```python
from build123d import *

# Parameters (mm, degrees)
F1_DEPTH  = 35
F2_R      = 3
F3_DEPTH  = 34.3740698971
F4_R      = 5
F5_DEPTH  = 120.001
F6_R      = 11.25
F7_DEPTH  = 7.5
F8_R      = 11.25
F9_DEPTH  = 7.5
F10_R     = 11.25
F11_DEPTH = 47.5
F12_R     = 11.25
F13_DEPTH = 47.5
F14_R     = 2.05
F15_DEPTH = 60
F16_R     = 3.5
F17_DEPTH = 15
F18_R     = 5


with BuildPart() as f1:
    # F0 (on Front) → F1 (new body)
    with BuildSketch(Plane.XZ):
        with BuildLine():
            Line((-40, 19.3730698971), (-60, 5))
            Line((-60, 5), (-60, 0))
            Line((-60, 0), (-60, -100))
            Line((-60, -100), (-40, -100))
            Line((-40, -100), (-30, -15))
            Line((-30, -15), (0, -15))
            Line((0, -15), (30, -15))
            Line((30, -15), (40, -100))
            Line((40, -100), (60, -100))
            Line((60, -100), (60, 0))
            Line((60, 0), (60, 5))
            Line((60, 5), (40, 19.3730698971))
            Line((40, 19.3730698971), (10, 19.3730698971))
            ThreePointArc((10, 19.3730698971), (0, 9.3730698971), (-10, 19.3730698971))
            Line((-10, 19.3730698971), (-40, 19.3730698971))
        make_face()
    extrude(amount=F1_DEPTH)

    # F2 (on face) → F3 (cut, through all)
    with BuildSketch(Plane(origin=(0, 0, -15), x_dir=(1, 0, 0), z_dir=(0, 0, -1))):
        with Locations((-16.9, 17.5)):
            Circle(F2_R)
        with Locations((16.9, 17.5)):
            Circle(F2_R)
    extrude(amount=-F3_DEPTH, mode=Mode.SUBTRACT)

    # F4 (on face) → F5 (cut, through all)
    with BuildSketch(Plane(origin=(-60, 0, 0), x_dir=(0, -1, 0), z_dir=(-1, 0, 0))):
        with Locations((17.5, -85)):
            Circle(F4_R)
    extrude(amount=-F5_DEPTH, mode=Mode.SUBTRACT)

    # F6 (on face) → F7 (cut)
    with BuildSketch(Plane(origin=(-60, 0, 0), x_dir=(0, -1, 0), z_dir=(-1, 0, 0))):
        with Locations((17.5, -85)):
            Circle(F6_R)
    extrude(amount=-F7_DEPTH, mode=Mode.SUBTRACT)

    # F8 (on face) → F9 (cut)
    with BuildSketch(Plane.YZ.offset(60)):
        with Locations((-17.5, -85)):
            Circle(F8_R)
    extrude(amount=-F9_DEPTH, mode=Mode.SUBTRACT)

    # F10 (on Right) → F11 (cut)
    with BuildSketch(Plane.YZ):
        with Locations((-17.5, -85)):
            Circle(F10_R)
    extrude(amount=-F11_DEPTH, mode=Mode.SUBTRACT)

    # F12 (on Right) → F13 (cut)
    with BuildSketch(Plane.YZ):
        with Locations((-17.5, -85)):
            Circle(F12_R)
    extrude(amount=F13_DEPTH, mode=Mode.SUBTRACT)

    # F14 (on Top) → F15 (cut, symmetric)
    with BuildSketch(Plane.XY):
        with Locations((-47, -18)):
            Circle(F14_R)
        with Locations((47, -18)):
            Circle(F14_R)
    extrude(amount=F15_DEPTH, both=True, mode=Mode.SUBTRACT)

    # F16 (on face) → F17 (cut)
    with BuildSketch(Plane.XY.offset(19.3730698971)):
        with Locations((-47, -18)):
            Circle(F16_R)
        with Locations((47, -18)):
            Circle(F16_R)
    extrude(amount=-F17_DEPTH, mode=Mode.SUBTRACT)

    # F18
    f18_edges = [f1.edges().sort_by_distance(p)[0] for p in [
        (60, -35, -47.5),
        (60, 0, -47.5),
        (-60, -35, -47.5),
        (-60, 0, -47.5),
        (-50, 0, 12.186535),
        (-50, -35, 12.186535),
        (50, -35, 12.186535),
        (50, 0, 12.186535),
        (35, 0, -57.5),
        (0, 0, -15),
        (0, -35, -15),
        (-35, -35, -57.5),
        (35, -35, -57.5),
        (-35, 0, -57.5),
    ]]
    fillet(f18_edges, radius=F18_R)


solid = f1.part
```
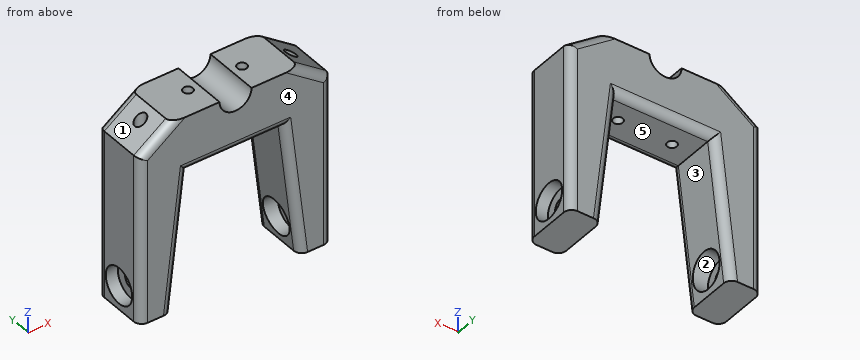
For this review, take the finished solid that the model builds, in its own axes (mm). Face numbers are marked on the shaded views. A direction names the side the tool comes from. Round coordinates to 2 decimals unless told otherwise and drop trailing zeros. Loops run counter-clockwise (first coordinate to the right, second up) from the corner with the lowest first, then second, coordinate; pieces in that order, holes last.
Q1. Add section A-A on x = 16.9. Write out the cut boundary in (y, z), plus the area to 3 significant figures.
Result sheet:
outline: (-35, -10) arc R5 ccw to (-30, -15) - (-20.5, -15) - (-20.5, 19.37) - (-35, 19.37) - close; (-14.5, -15) - (-5, -15) arc R5 ccw to (0, -10) - (0, 19.37) - (-14.5, 19.37) - close
area: 986 mm2
Q2. Add section C-C on y = -1.5. Write out the cut boundary in (x, z).
Result sheet:
outline: (-58.57, -100) - (-41.44, -100) - (-31.27, -13.57) - (31.27, -13.57) - (41.44, -100) - (58.57, -100) - (58.57, 4.27) - (37.55, 19.37) - (10, 19.37) arc R10 cw to (-10, 19.37) - (-37.55, 19.37) - (-58.57, 4.27) - close
Q3. Add section B-B on z = -30. Give the number of separate pieces and of enclosed holes in the cut face, plus the area to 3 significant figures.
Result sheet:
separate pieces: 2
enclosed holes: 2
area: 1,910 mm2
Q4. Insertion check: pin 1 Ø11.5 at (y, z) = (-17.5, -85) entering from +X; pin 2 Ø10 at (x, y) = (-46.5, -14) entering from +Z; pin 3 Ø11 at (y, z) = (-17, -81) entering from -X. Each pin has a flat end and moves straight along its axis. Give the tip position at first contact, or say it passes through.
Result sheet:
pin 1: stops at x = 52.5
pin 2: stops at z = 18.3
pin 3: stops at x = -52.5
Q5. Add section D-D on x = 0. Write out the cut boundary in (y, z), plus the area to 3 significant figures.
Result sheet:
outline: (-35, -10) arc R5 ccw to (-30, -15) - (-5, -15) arc R5 ccw to (0, -10) - (0, 9.37) - (-35, 9.37) - close
area: 842 mm2
Q6. Machinability: for the marked faces 4 and 5, which of the approach directions +Z, -Z, +X, -X, +Y, -Y give a long, thin tool a straight path to every point of the face, cutting with its end or side? Answer none if there is none.
Result sheet:
face 4: +Z, -Z, +X, -X, -Y
face 5: -Z, +Y, -Y
Q7. To check wall thickness, follow line 1 along Z through (x, y) = (48, -17); line 2 along Z through (x, y) = (10.5, -6); line 3 along X through (y, z) = (-17, -2). State the ranges of each line that lie inside material, in increasing order.
Result sheet:
line 1: z = -100 to -89.97, -80.03 to -60
line 2: z = -15 to 19.37
line 3: x = -60 to -48.79, -45.21 to -19.86, -13.94 to 13.94, 19.86 to 45.21, 48.79 to 60
Q8. Mouldability with a two-part tool opening along Z and no side actions: class the marked faces 1, 2 and 3 as +Z half, -Z half, draft (parallel to the pull), parting line (faces both ways), or undercut.
Result sheet:
face 1: +Z half
face 2: undercut
face 3: -Z half
